Design review of the part built by this model. Coordinates are the model's own, in mm. A direction names the side the tool comes from. Round coordinates to 2 decimals unless told otherwise and drop trailing zeros. Order: outer loops, then holes, each group sorted by start corner. A loop starts at its lowest first (then second) coordinate and runs counter-clockwise, first axis right, second up. Notation, with made-up numbers: (-26.5, 52) - (2.5, 52) arc R17 ccw to (2.5, 64) - close; hole circle Ø10 at (37, -11). An arc over 180 degrees is marked (long way). Use CSV: the item, a comma, the result in double quotes.
from build123d import *

# Parameters (mm, degrees)
F0_R     = 15.875
F1_DEPTH = 31.75
F2_R     = 19.05
F2_R_2   = 15.875
F3_DEPTH = 6.35
F5_R     = 12.065
F6_DEPTH = 63.501


with BuildPart() as f1:
    # F0 (on Front) → F1 (new body, symmetric)
    with BuildSketch(Plane.XZ):
        Circle(F0_R)
    extrude(amount=F1_DEPTH, both=True)

    # F2 (on face) → F3 (join)
    with BuildSketch(Plane.XZ.offset(31.75)):
        Circle(F2_R)
        Circle(F2_R_2, mode=Mode.SUBTRACT)
    extrude(amount=-F3_DEPTH)

    # F4: F1 across plane


with BuildPart() as f1_1:
    add(f1.part)
    add(f1.part.mirror(Plane.XZ))

    # F5 (on face) → F6 (cut, through all)
    with BuildSketch(Plane.XZ.offset(31.75)):
        Circle(F5_R)
    extrude(amount=-F6_DEPTH, mode=Mode.SUBTRACT)


solid = f1_1.part
1) We need section A-A (z = 0). Give the boundary of the cut face in (x, y) (3 decimals).
Data:
outline,"(-19.05, -31.75) - (-12.065, -31.75) - (-12.065, 31.75) - (-19.05, 31.75) - (-19.05, 25.4) - (-15.875, 25.4) - (-15.875, -25.4) - (-19.05, -25.4) - close; (12.065, -31.75) - (19.05, -31.75) - (19.05, -25.4) - (15.875, -25.4) - (15.875, 25.4) - (19.05, 25.4) - (19.05, 31.75) - (12.065, 31.75) - close"
2) To check wall thickness, follow L1, parallel to Z at x = 0, y = -10 (3 decimals); L2, parallel to Y at x = 14, z = -8; L3, parallel to X at y = -21.5, z = -4.5. State the ranges of each line that lie inside material, in increasing order. Write a range as from..to.
Data:
L1,"z = -15.875..-12.065, 12.065..15.875"
L2,"y = -31.75..-25.4, 25.4..31.75"
L3,"x = -15.22..-11.19, 11.19..15.22"
3) We need section B-B (x = -9). Give the boundary of the cut face in (y, z).
Data:
outline,"(-31.75, -16.79) - (-25.4, -16.79) - (-25.4, -13.08) - (25.4, -13.08) - (25.4, -16.79) - (31.75, -16.79) - (31.75, -8.04) - (-31.75, -8.04) - close; (-31.75, 8.04) - (31.75, 8.04) - (31.75, 16.79) - (25.4, 16.79) - (25.4, 13.08) - (-25.4, 13.08) - (-25.4, 16.79) - (-31.75, 16.79) - close"
4) We need section C-C (y = 22.5). Give the boundary of the cut face in (x, z) (3 decimals).
Data:
outline,"circle Ø31.75 at (0, 0); hole circle Ø24.13 at (0, 0)"
5) For faces 1 (the face through (-3.441, -0.356, -15.497)), 2 (the face through (-0.3, 31.75, -12.4)), list the 3-axis set-ups (+Z, -Z, +X, -X, +Y, -Y) from which the entire face can be reached by the end or side of a thin tool; tool diameter is ignored.
Data:
face 1,"none"
face 2,"+Z, -Z, +X, -X, +Y"
6) The part is to be moulded in two halves that separate along Y. For faces 3 (the face through (-15.12, -28.62, -11.59)), 4 (the face through (-0.3, -31.75, -12.4)), 5 (the face through (-4, -25.4, 16)), say which applies: +Y half, -Y half, draft (parallel to the pull), parting line (faces both ways), or undercut.
Data:
face 3,"draft"
face 4,"-Y half"
face 5,"undercut"
7) Insertion check: pin 1 Ø4 at (x, y) = (-5, 17.5) entering from -Z; pin 2 Ø12 at (x, y) = (12.5, 16.5) entering from -Z; pin 3 Ø1.5 at (y, z) = (24.5, -9.5) entering from +X. Each pin has a flat end and moves straight along its axis. Give the tip position at first contact, or say it passes through.
Data:
pin 1,"stops at z = -15.59"
pin 2,"stops at z = -14.48"
pin 3,"stops at x = 13.25"
